```python
from build123d import *

# Parameters (mm, degrees)
F0_R     = 46
F0_R_2   = 43.5
F1_DEPTH = 2
F0_R_3   = 49
F2_DEPTH = 4
F0_R_4   = 51
F3_DEPTH = 12
F4_R     = 1
F5_SIZE2 = 3
F5_SIZE  = 6
F6_R     = 2


with BuildPart() as f1:
    # F0 (on Top) → F1 (new body)
    with BuildSketch(Plane.XY):
        Circle(F0_R)
        Circle(F0_R_2, mode=Mode.SUBTRACT)
    extrude(amount=F1_DEPTH)

    # F0 (on Top) → F2 (join)
    with BuildSketch(Plane.XY):
        Circle(F0_R_3)
        Circle(F0_R, mode=Mode.SUBTRACT)
    extrude(amount=F2_DEPTH)

    # F0 (on Top) → F3 (join)
    with BuildSketch(Plane.XY):
        Circle(F0_R_4)
        Circle(F0_R_3, mode=Mode.SUBTRACT)
    extrude(amount=F3_DEPTH)

    # F4
    f4_edges = [f1.edges().sort_by_distance(p)[0] for p in [
        (-43.5, 0, 2),
        (-46, 0, 4),
    ]]
    fillet(f4_edges, radius=F4_R)

    # F5
    f5_edges = [f1.edges().sort_by_distance(p)[0] for p in [
        (-51, 0, 0),
    ]]
    f5_side = f1.faces().sort_by_distance((-51, 0, 6))[0]
    chamfer(f5_edges, length=F5_SIZE, length2=F5_SIZE2, reference=f5_side)

    # F6
    f6_edges = [f1.edges().sort_by_distance(p)[0] for p in [
        (-51, 0, 6),
        (49.5, 0, 3),
        (-48, 0, 0),
    ]]
    fillet(f6_edges, radius=F6_R)


solid = f1.part
```
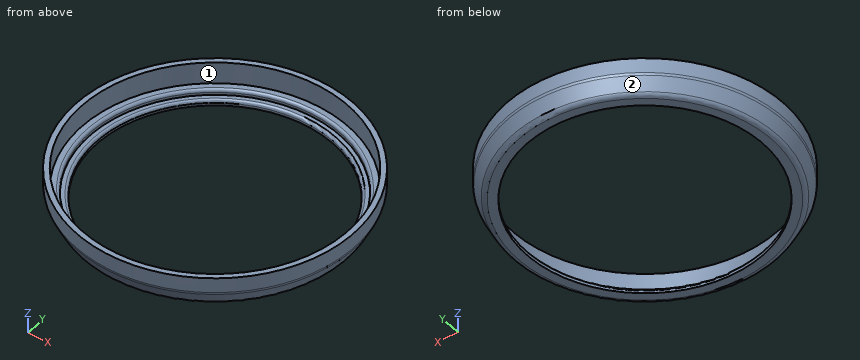
Could you check a few things on this model? Use its own coordinates, in mm. Face numbers are marked on the shaded views. Round coordinates to 2 decimals unless told otherwise and drop trailing zeros.
(1) For pin 1 (2 mm diameter, centred on x = 7, z = 5, fed in from +Y); pin 2 (2 mm diameter, centred on x = -22, y = -38, fed in from +Z); pin 3 (6 mm diameter, centred on y = -21.5, z = 4.5, fed in from +X), each with a flat end and sliding along its axis, tell me the tip position at first contact or that it passes through.
Findings below:
pin 1: stops at y = 50.49
pin 2: stops at z = 2
pin 3: stops at x = 47.31
(2) If I drill on probe 1 along X at (y, z) = (33.5, 3.5); probe 2 along Y at (x, z) = (-2, 1); probe 3 along X at (y, z) = (-37, 1.75), over which ranges is the centre line in solid material (lowest first)?
Findings below:
probe 1: x = -36.78 to -31.72, 31.72 to 36.78
probe 2: y = -48.45 to -43.45, 43.45 to 48.45
probe 3: x = -31.93 to -23.51, 23.51 to 31.93
(3) Thinking about a two-plate mould opening in Y: for the marked faces 1 and 2, which applies, +Y half, -Y half, draft (parallel to the pull), parting line (faces both ways), or undercut?
Findings below:
face 1: undercut
face 2: parting line
